from build123d import *

# Parameters (mm, degrees)
BOSS_EXTRUDE1_DEPTH = 1
SKETCH2_R           = 1.9
SKETCH2_W           = 9.8
SKETCH2_H           = 29.28075205
BOSS_EXTRUDE2_DEPTH = 0.5
FILLET1_R           = 1
BOSS_EXTRUDE3_START = -1
BOSS_EXTRUDE3_DEPTH = 1


with BuildPart() as part:
    # Sketch1 → Boss-Extrude1 (new body)
    with BuildSketch(Plane(origin=(0, 0, 0), x_dir=(1, 0, 0), z_dir=(0, 1, 0))):
        with BuildLine():
            Line((-21.771541057, 7.1), (-1.980475175, 7.1))
            Line((-1.980475175, 7.1), (-1.980475175, -7.1))
            Line((-1.980475175, -7.1), (-21.771541057, -7.1))
            ThreePointArc((-21.771541057, -7.1), (22.9, 0), (-21.771541057, 7.1))
        make_face()
    extrude(amount=BOSS_EXTRUDE1_DEPTH)

    # Sketch2 → Boss-Extrude2 (add)
    with BuildSketch(Plane.XZ):
        with Locations(Location((-11.642490831, 11, 0), (0, 0, 90))):
            Circle(SKETCH2_R)
        with Locations(Location((-11.642490831, -11, 0), (0, 0, 90))):
            Circle(SKETCH2_R)
        with Locations((10, 0)):
            Rectangle(SKETCH2_W, SKETCH2_H)
    extrude(amount=BOSS_EXTRUDE2_DEPTH)

    # Fillet1
    fillet1_edges = [part.edges().sort_by_distance(p)[0] for p in [
        (-1.980475175, 1, 0),
    ]]
    fillet(fillet1_edges, radius=FILLET1_R - 0.0001)  # a hair under: the kernel refuses the full size

    # Sketch3 → Boss-Extrude3 (add)
    with BuildSketch(Plane(origin=(0, 1, 0), x_dir=(1, 0, 0), z_dir=(0, 1, 0)).offset(BOSS_EXTRUDE3_START)):
        with BuildLine():
            Line((-6.980475175, -7.1), (-21.771541057, -7.1))
            ThreePointArc((-21.771541057, -7.1), (-22.9, 0), (-21.771541057, 7.1))
            Line((-21.771541057, 7.1), (-6.980475175, 7.1))
            Line((-6.980475175, 7.1), (-6.980475175, -7.1))
        make_face()
    extrude(amount=BOSS_EXTRUDE3_DEPTH)


solid = part.part
Build history of the part. All positions in model axes, mm. A direction names the side the tool comes from. Round coordinates to 2 decimals unless told otherwise and drop trailing zeros. Write each loop counter-clockwise with the first axis right and the second up, starting at its lowest first coordinate (ties: lowest second). Pieces come first, ordered by that corner, then holes. Notation, with made-up numbers: M 66.5,-7.75 L 82.5,-7.75 A23 ccw 82.5,28.25 Z; hole C 74,33.25 d5. An arc over 180 degrees is marked long. Answer as a JSON object with one key per item and string values. Group by question number.
(1) Cut at D-D (x = 0). Give the cut face in (y, z), and give its area (3 significant figures).
(2) Which spindle directions (+Z, -Z, +X, -X, +Y, -Y) get a long thin tool onto all of the face, cutting with end or side? Do faces 1 (the cylindrical face through (-13.245, -0.246, -9.979)), 2 (the flat face through (-6.98, 0.5, -0.1)), 3 (the flat face through (10, -0.5, 0)). Say none if no direction does.
(3) Mould opens along Z. For faces 4 (the cylindrical face through (-1.695, 0.699, 0.099)), 5 (the flat face through (0, 1, 0)) say: pulls with the +Z half, pulls with the -Z half, needs draft (parallel to the pull), parting line crosses it, or undercut.
(4) Flat gauge pins, fed straight in: pin 1 (0.6 mm diameter, centred on y = 0, z = 6.5, fed in from +X); pin 2 (0.8 mm diameter, centred on y = 0.5, z = 2, fed in from +X); pin 3 (0.8 mm diameter, centred on x = -3, y = 0.5, fed in from -Z). Where does each tip first touch, or does it go through?
(5) Cut at B-B (y = 0.3). Give the cut face in (x, z).
(6) Drill centre lines: L1, parallel to Y at x = 1, z = -2.5; L2, parallel to X at y = -0.25, z = -2; L3, parallel to X at y = 0.6, z = 6.5. Where is each one in solid material? Low to high.
Responses:
{
 "1": {"outline": "M 0,-22.9 L 1,-22.9 L 1,22.9 L 0,22.9 Z", "area": "45.8 mm2"},
 "2": {"face 1": "-Y", "face 2": "+Y, -Y", "face 3": "+Z, -Z, +X, -X, -Y"},
 "3": {"face 4": "undercut", "face 5": "needs draft"},
 "4": {"pin 1": "stops at x = 22.04", "pin 2": "stops at x = 22.84", "pin 3": "stops at z = -22.75"},
 "5": {"outline": "C 0,0 d45.8; hole M -6.98,-7.1 L -1.93,-7.1 L -1.93,7.1 L -6.98,7.1 Z"},
 "6": {"L1": "y = 0 to 1", "L2": "x = 5.1 to 14.9", "L3": "x = -21.96 to -6.98, -1.78 to 21.96"}
}
